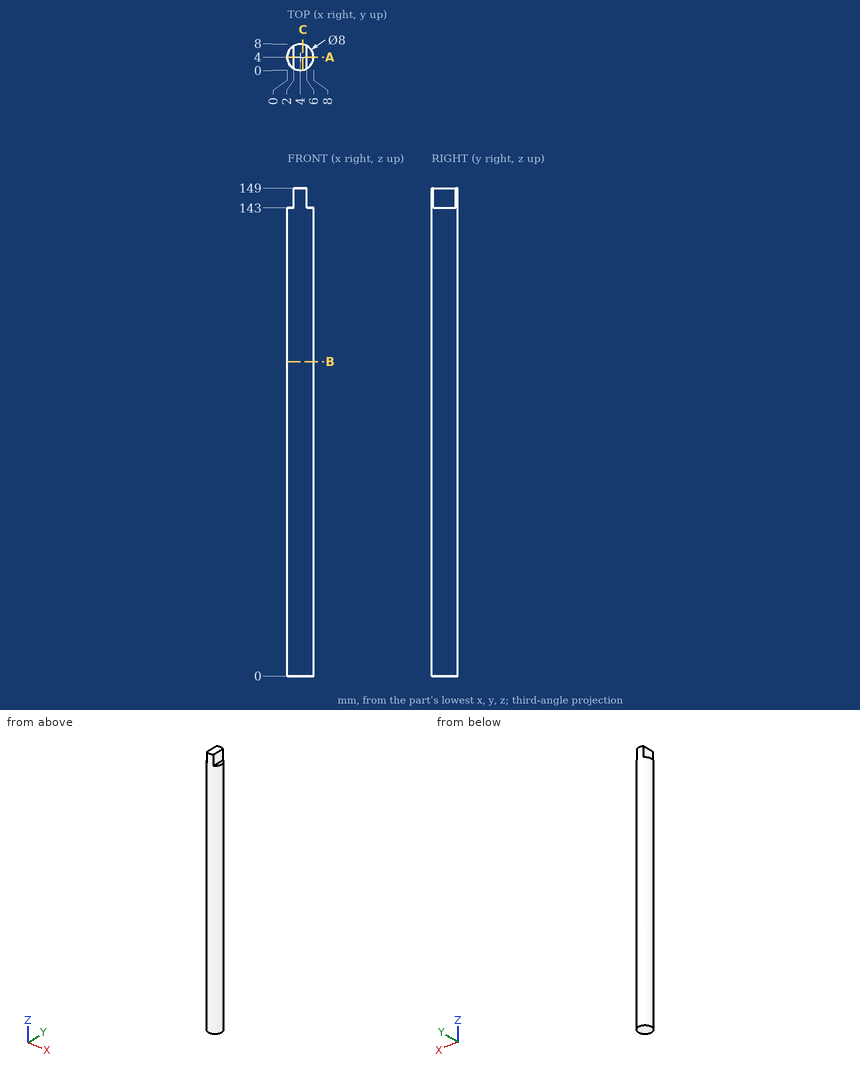
Check sheet for the drawn part. Datum: minimum x, y, z corner. Units: mm. Give positions to 0.01 mm unless a question says otherwise; leave off trailing zeros. Order: outer loops, then holes, each group sorted by start corner. A loop starts at its lowest first (then second) coordinate and runs counter-clockwise, first axis right, second up. Notation, with made-up numbers: (43.25, 6.25) -> (81.25, 6.25) arc R19 cw to (81.25, 28.25) -> close; hole circle Ø1 at (82.25, 88.25). An arc over 180 degrees is marked (long way). Use a Markdown table: item, result.
1) Section check C-C, the plane x = 4.75. Record the boundary of the cut face in (y, z), then the cut area to 3 significant figures.
Results:
| item | result |
|---|---|
| outline | (0.07, 0) -> (7.93, 0) -> (7.93, 149) -> (0.07, 149) -> close |
| area | 1,170 mm² |
2) Material ranges on probe 1 along Z at (x, y) = (6.5, 6.5); probe 2 along X at (y, z) = (6, 142.5); probe 3 along X at (y, z) = (7.5, 129), recorded low to high.
Results:
| item | result |
|---|---|
| probe 1 | 0 to 143 |
| probe 2 | 0.54 to 7.46 |
| probe 3 | 2.06 to 5.94 |
3) Section check B-B, the plane z = 96. Record the boundary of the cut face in (x, y), then the cut area to 3 significant figures.
Results:
| item | result |
|---|---|
| outline | circle Ø8 at (4, 4) |
| area | 50.3 mm² |
4) Depth check by flat-ended pin: pin 1 Ø1 at (x, z) = (2.5, 30) entering from +Y; pin 2 Ø1.5 at (x, z) = (6.5, 22) entering from +Y; pin 3 Ø1 at (x, y) = (0.5, 3) entering from +Z. Enter the tip coordinate at first touch or a pass-through.
Results:
| item | result |
|---|---|
| pin 1 | y = 7.87 |
| pin 2 | y = 7.6 |
| pin 3 | z = 143 |
5) Section check A-A, the plane y = 4. Record the boundary of the cut face in (x, z).
Results:
| item | result |
|---|---|
| outline | (0, 0) -> (8, 0) -> (8, 143) -> (6, 143) -> (6, 149) -> (2, 149) -> (2, 143) -> (0, 143) -> close |
